Verification items for the finished model (mm, model axes). A direction names the side the tool comes from. Give positions to 0.01 mm unless a question says otherwise; leave off trailing zeros. Write each loop counter-clockwise with the first axis right and the second up, starting at its lowest first coordinate (ties: lowest second). Pieces come first, ordered by that corner, then holes. Notation, with made-up numbers: (29, 1.5) - (41, 1.5) arc R15 ccw to (41, 27.5) - close; hole circle Ø2 at (89, 19.5). An arc over 180 degrees is marked (long way). Answer as a JSON object with one key per item and string values. Group by question number.
Item 1: Sectioned sample at C-C, the plane z = 4. Record the boundary of the cut face in (x, y).
Item 2: Go/stop test with flat-tipped pins: pin 1 (4 mm diameter, centred on y = -3.5, z = 8, fed in from -X); pin 2 (1.5 mm diameter, centred on y = 4.5, z = 7.5, fed in from +X). Record where each tip stops, or that it passes through.
Item 3: Tool access check on faces 1 (the face through (1, -2, 0)), 2 (the face through (-3, 5, 8)). Record the directions out of +Z, -Z, +X, -X, +Y, -Y that give a thin tool (end or side, any length) a straight path to the whole face; none if there is none.
Item 4: Scan lines: line 1 along Y through (x, z) = (0, 2.4); line 2 along Z through (x, y) = (-7.25, 3.75); line 3 along X through (y, z) = (1, 0.5). Record each from-to range of solid material in increasing order. Write a range as [from, to].
Item 5: Draft check along X on faces 3 (the face through (0, 2, 2)), 4 (the face through (-1.19, -5.37, 7.49)), 5 (the face through (0, 0, 9.5)). Enter one of: +X half, -X half, draft (parallel to the pull), parting line (faces both ways), or undercut.
Item 6: Sectioned sample at A-A, the plane y = 0. Record the boundary of the cut face in (x, z), and give its area (3 significant figures).
```python
from build123d import *

# Parameters (mm, degrees)
F0_R     = 4
F1_DEPTH = 7
F2_R     = 5.5
F2_R_2   = 4
F3_DEPTH = 1
F4_R     = 11
F5_DEPTH = 1.5
F6_R     = 2
F7_DEPTH = 5
F8_SIZE  = 1
F9_SIZE  = 1


with BuildPart() as f1:
    # F0 (on Top) → F1 (new body)
    with BuildSketch(Plane.XY):
        Circle(F0_R)
    extrude(amount=F1_DEPTH)

    # F2 (on face) → F3 (join)
    with BuildSketch(Plane.XY.offset(7)):
        Circle(F2_R)
        Circle(F2_R_2, mode=Mode.SUBTRACT)
        Circle(F2_R_2)
    extrude(amount=F3_DEPTH)

    # F4 (on face) → F5 (join)
    with BuildSketch(Plane.XY.offset(8)):
        Circle(F4_R)
    extrude(amount=F5_DEPTH)

    # F6 (on face) → F7 (cut)
    with BuildSketch(Plane(origin=(0, 0, 0), x_dir=(1, 0, 0), z_dir=(0, 0, -1))):
        Circle(F6_R)
    extrude(amount=-F7_DEPTH, mode=Mode.SUBTRACT)

    # F8
    f8_edges = [f1.edges().sort_by_distance(p)[0] for p in [
        (-4, 0, 0),
    ]]
    chamfer(f8_edges, length=F8_SIZE)

    # F9
    f9_edges = [f1.edges().sort_by_distance(p)[0] for p in [
        (-11, 0, 9.5),
    ]]
    chamfer(f9_edges, length=F9_SIZE)


solid = f1.part
```
Geometry check:
{
 "1": {"outline": "circle Ø8 at (0, 0); hole circle Ø4 at (0, 0)"},
 "2": {"pin 1": "x = -10.9", "pin 2": "x = 10.27"},
 "3": {"face 1": "-Z, +X, -X, +Y, -Y", "face 2": "-Z"},
 "4": {"line 1": "[-4, -2], [2, 4]", "line 2": "[8, 9.5]", "line 3": "[-3.35, -1.73], [1.73, 3.35]"},
 "5": {"face 3": "undercut", "face 4": "parting line", "face 5": "draft"},
 "6": {"outline": "(-11, 8) - (-5.5, 8) - (-5.5, 7) - (-4, 7) - (-4, 1) - (-3, 0) - (-2, 0) - (-2, 5) - (2, 5) - (2, 0) - (3, 0) - (4, 1) - (4, 7) - (5.5, 7) - (5.5, 8) - (11, 8) - (11, 8.5) - (10, 9.5) - (-10, 9.5) - (-11, 8.5) - close", "area": "78.0 mm^2"}
}
